Here's the drawing with two shaded views (mm, measured from the low corner). I have some questions. Give positions to 0.01 mm unless a question says otherwise; leave off trailing zeros. Loops run counter-clockwise (first coordinate to the right, second up) from the corner with the lowest first, then second, coordinate; pieces in that order, holes last. Notation, with made-up numbers: (48.25, -22.5) - (60.25, -22.5) arc R10 cw to (60.25, -11.5) - close; hole circle Ø2 at (65.25, 8.5). An arc over 180 degrees is marked (long way). Answer as a JSON object with one key per item and string values. Group by question number.
Item 1: Please list where these lines run through material, in increasing order: L1, parallel to X at y = 26.5, z = 27 (1 decimal); L2, parallel to Y at x = 59.5, z = 32; L3, parallel to Y at x = 46, z = 15.
Item 2: Suppose I cut it at C-C on y = 45. Write out the boundary of the cut face in (x, z), and give its area (3 significant figures).
Item 3: Thinking about a two-plate mould opening in Y: for the marked faces 1, 2, 3 and 4, which applies, pulls with the +Y half, pulls with the -Y half, needs draft (parallel to the pull), parting line crosses it, or undercut?
Item 4: Will these pins go through, and if not, where does the flat tip stop? pin 1 (1.7 mm diameter, centred on y = 45, z = 29.5, fed in from -X) (1 decimal); pin 2 (1 mm diameter, centred on y = 43, z = 18.5, fed in from +X); pin 3 (1.5 mm diameter, centred on y = 42, z = 26, fed in from +X) (1 decimal).
Item 5: Suppose I cut it at D-D on z = 34. Write out the boundary of the cut face in (x, y), and give its area (3 significant figures).
Item 6: Suppose I cut it at A-A on x = 32.5. Write out the boundary of the cut face in (y, z) (1 decimal).
Item 7: Suppose I cut it at B-B on y = 25. Write out the boundary of the cut face in (x, z) (1 decimal), and give its area (3 significant figures).
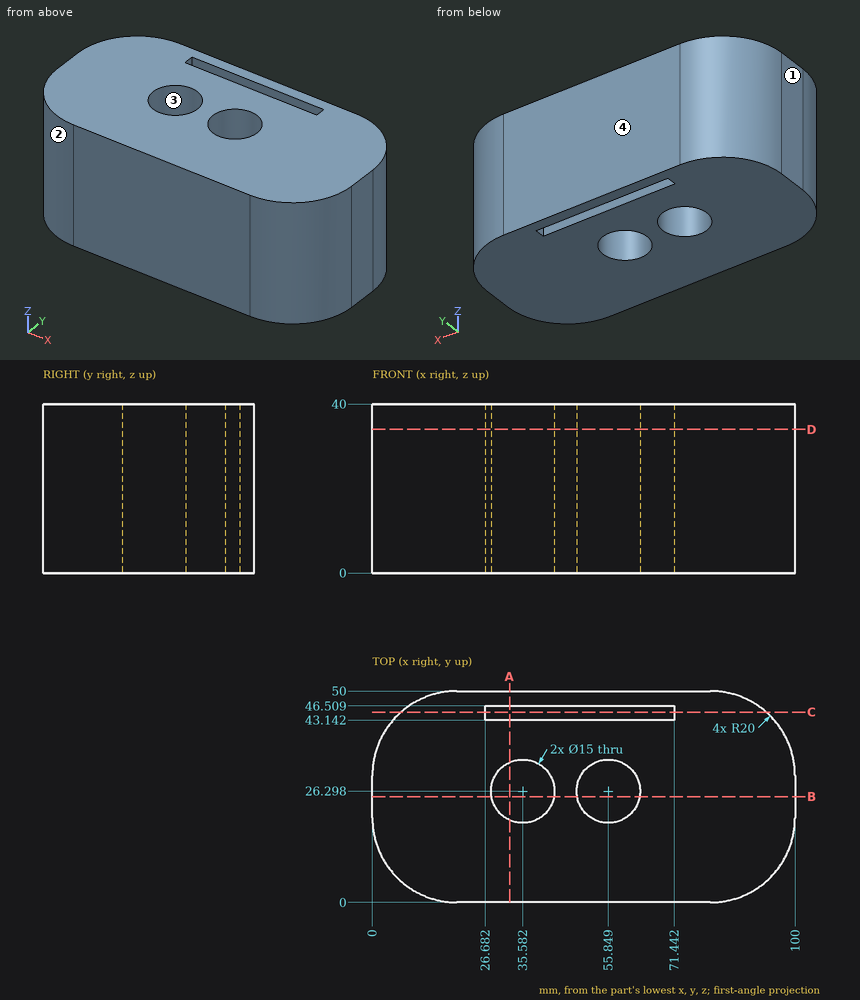
Worked out:
{
 "1": {"L1": "x = 0 to 28.1, 43.1 to 48.4, 63.3 to 100", "L2": "y = 0 to 19.75, 32.85 to 43.14, 46.51 to 50", "L3": "y = 0 to 43.14, 46.51 to 50"},
 "2": {"outline": "(6.77, 0) - (26.68, 0) - (26.68, 40) - (6.77, 40) - close; (71.44, 0) - (93.23, 0) - (93.23, 40) - (71.44, 40) - close", "area": "1,670 mm2"},
 "3": {"face 1": "needs draft", "face 2": "pulls with the -Y half", "face 3": "undercut", "face 4": "pulls with the +Y half"},
 "4": {"pin 1": "stops at x = 5.9", "pin 2": "stops at x = 95.61", "pin 3": "stops at x = 96.5"},
 "5": {"outline": "(0, 20) arc R20 ccw to (20, 0) - (80, 0) arc R20 ccw to (100, 20) - (100, 30) arc R20 ccw to (80, 50) - (20, 50) arc R20 ccw to (0, 30) - close; hole (26.68, 43.14) - (71.44, 43.14) - (71.44, 46.51) - (26.68, 46.51) - close; hole circle Ø15 at (35.58, 26.3); hole circle Ø15 at (55.85, 26.3)", "area": "4,150 mm2"},
 "6": {"outline": "(0, 0) - (19.5, 0) - (19.5, 40) - (0, 40) - close; (33.1, 0) - (43.1, 0) - (43.1, 40) - (33.1, 40) - close; (46.5, 0) - (50, 0) - (50, 40) - (46.5, 40) - close"},
 "7": {"outline": "(0, 0) - (28.2, 0) - (28.2, 40) - (0, 40) - close; (43, 0) - (48.5, 0) - (48.5, 40) - (43, 40) - close; (63.2, 0) - (100, 0) - (100, 40) - (63.2, 40) - close", "area": "2,820 mm2"}
}
